CAD build for the part. Positions are in the model's coordinates, mm. A direction names the side the tool comes from. Round coordinates to 2 decimals unless told otherwise and drop trailing zeros. Write each loop counter-clockwise with the first axis right and the second up, starting at its lowest first coordinate (ties: lowest second). Pieces come first, ordered by that corner, then holes. Notation, with made-up numbers: (-33, 45) -> (-16, 45) arc R7 ccw to (-16, 53) -> close; hole circle Ø3 at (-3.5, 39.25). An arc over 180 degrees is marked (long way). Answer in a Markdown table with one row per item. Add a question column.
```python
from build123d import *

# Parameters (mm, degrees)
EXTRUDE_1_DEPTH          = 10
PATTERN_CIRCULAR_1_COUNT = 55
EXTRUDE_START            = -6
EXTRUDE_2_DEPTH          = 6
SKETCH_4_R               = 7
CUT_EXTRUDE_1_DEPTH      = 0.5
FILLET_2_R               = 0.5


with BuildPart() as part:
    # Эскиз1 → Повернуть1 (revolve)
    with BuildSketch(Plane.XY, mode=Mode.PRIVATE) as revolve_1_sk:
        Polygon((-5, 17), (-4.5, 17), (-4.5, 12), (-2.5, 12), (-2.5, 0), (-5, 0), (-5, 10), (-8.5, 10), (-8.5, 11.5), align=None)
    revolve(revolve_1_sk.sketch.rotate(Axis((0, -50, 0), (0, 1, 0)), 270), axis=Axis((0, -50, 0), (0, 1, 0)))

    # Эскиз2 → Бобышка-Вытянуть1 (add)
    with BuildSketch(Plane.XZ):
        Polygon((-0.25, 4.399667297), (0, 5.5), (0.25, 4.399667297), align=None)
    extrude_1 = extrude(amount=-EXTRUDE_1_DEPTH)

    # Круговой массив1: Бобышка-Вытянуть1 ×55 about axis
    pattern_circular_1_axis = Axis((0, 0, 0), (0, 1, 0))
    for i in range(1, PATTERN_CIRCULAR_1_COUNT):
        add(extrude_1.rotate(pattern_circular_1_axis, i * 360 / PATTERN_CIRCULAR_1_COUNT))

    # Эскиз3 → Бобышка-Вытянуть2 (add)
    with BuildSketch(Plane(origin=(0, 17, 0), x_dir=(1, 0, 0), z_dir=(0, 1, 0)).offset(EXTRUDE_START)):
        with BuildLine():
            Line((-1.479019946, 4.25), (1.479019946, 4.25))
            ThreePointArc((1.479019946, 4.25), (0, 4.5), (-1.479019946, 4.25))
        make_face()
        with BuildLine():
            Line((-1.479019946, -4.25), (1.479019946, -4.25))
            ThreePointArc((1.479019946, -4.25), (0, -4.5), (-1.479019946, -4.25))
        make_face()
    extrude(amount=EXTRUDE_2_DEPTH)

    # Эскиз4 → Вырез-Вытянуть1 (cut)
    with BuildSketch(Plane(origin=(0, 17, 0), x_dir=(1, 0, 0), z_dir=(0, 1, 0))):
        Circle(SKETCH_4_R)
    extrude(amount=-CUT_EXTRUDE_1_DEPTH, mode=Mode.SUBTRACT)

    # Скругление2
    fillet_2_edges = [part.edges().sort_by_distance(p)[0] for p in [
        (0, 16.5, 5.318181818),
    ]]
    fillet(fillet_2_edges, radius=FILLET_2_R)


solid = part.part
```
Item 1: Saw through at A-A on y = 14. Give the cut face in (x, z).
Item 2: Pin check, flat tips, straight feed: pin 1 (3 mm diameter, centred on x = 2.5, y = 14, fed in from +Z); pin 2 (3 mm diameter, centred on y = 3, z = -5.5, fed in from -X); pin 3 (1.5 mm diameter, centred on y = 12.5, z = 3, fed in from +X). Stop position of each tip, or through.
Item 3: Two-plate mould, pull along X, no slides. Class faces 1 (the cylindrical face through (-8.428, 10.76, 1.107)), 2 (the flat face through (0, 14, 4.25)), 3 (the flat face through (-0.4, 16.5, 4.5)): +X half, -X half, draft (parallel to the pull), parting line (faces both ways), or undercut.
Item 4: Tool access for faces 4 (the flat face through (0, 14, -4.25)), 5 (the cylindrical face through (2.44, 5.92, 0.54)): list every direction of +Z, -Z, +X, -X, +Y, -Y with a clear straight run to the whole face (end or side of a thin tool).
Item 5: Drill centre lines: probe 1 along X at (y, z) = (7, 0); probe 2 along Z at (x, y) = (-6.5, 12.25); probe 3 along Z at (x, y) = (-0.5, 13). Where is each one in solid material? Low to high.
Recorded:
| question | item | result |
|---|---|---|
| 1 | outline | circle Ø13.82 at (0, 0); hole (-1.48, -4.25) -> (1.48, -4.25) arc R4.5 ccw to (1.48, 4.25) -> (-1.48, 4.25) arc R4.5 ccw to start |
| 2 | pin 1 | z = 7.55 |
| 2 | pin 2 | x = -3.72 |
| 2 | pin 3 | x = 7.85 |
| 3 | face 1 | parting line |
| 3 | face 2 | undercut |
| 3 | face 3 | draft |
| 4 | face 4 | +Y |
| 4 | face 5 | +Y, -Y |
| 5 | probe 1 | -5 to -2.5, 2.5 to 5 |
| 5 | probe 2 | -4.7 to 4.7 |
| 5 | probe 3 | -7.53 to -4.25, 4.25 to 7.53 |
